For this review, take the finished solid that the model builds, in its own axes (mm). A direction names the side the tool comes from. Coordinates: 2 decimals unless noted, no trailing zeros. Loops run counter-clockwise (first coordinate to the right, second up) from the corner with the lowest first, then second, coordinate; pieces in that order, holes last. Notation, with made-up numbers: (24.5, 18.5) -> (60.5, 18.5) arc R3 ccw to (60.5, 23.5) -> close; hole circle Ø1 at (12, 62.25). An arc over 180 degrees is marked (long way). Use a Markdown table: item, result.
from build123d import *

# Parameters (mm, degrees)
SKETCH1_W            = 20
SKETCH1_H            = 28.7
BOSS_EXTRUDE1_DEPTH  = 17.15
CUT_EXTRUDE1_START   = -1.56
SKETCH2_R            = 7.85
CUT_EXTRUDE1_DEPTH   = 25.58
CUT_EXTRUDE2_DEPTH   = 39.959113
BOSS_EXTRUDE2_DEPTH  = 6.3
M4_CLEARANCE_HOLE1_D = 4.8
CUT_REVOLVE3_START   = -16.206498
CUT_REVOLVE3_DEPTH   = 3.8
CUT_REVOLVE4_START   = -16.206498
CUT_REVOLVE4_DEPTH   = 3.8
SKETCH10_W           = 20
SKETCH10_H           = 3.8
CUT_EXTRUDE3_DEPTH   = 5.3
FILLET1_R            = 2


# Read off the part's stored shape, not the designer's step: Cut-Revolve3, Cut-Revolve4
with BuildPart() as part:
    # Sketch1 → Boss-Extrude1 (new body)
    with BuildSketch(Plane(origin=(0, 0, 0), x_dir=(1, 0, 0), z_dir=(0, 1, 0))):
        with Locations((10, 14.35)):
            Rectangle(SKETCH1_W, SKETCH1_H)
    extrude(amount=BOSS_EXTRUDE1_DEPTH)

    # Sketch2 → Cut-Extrude1 (cut)
    with BuildSketch(Plane.XY.offset(CUT_EXTRUDE1_START)):
        with Locations((10, 17.15)):
            Circle(SKETCH2_R)
    extrude(amount=-CUT_EXTRUDE1_DEPTH, mode=Mode.SUBTRACT)

    # Sketch3 → Cut-Extrude2 (cut, through all)
    with BuildSketch(Plane.XY):
        with BuildLine():
            Line((2.15, 17.15), (17.85, 17.15))
            ThreePointArc((17.85, 17.15), (17.260735, 14.166005), (15.581407, 11.63))
            Line((15.581407, 11.63), (14.85, 11.63))
            Line((14.85, 11.63), (5.15, 11.63))
            Line((5.15, 11.63), (4.418593, 11.63))
            ThreePointArc((4.418593, 11.63), (2.739265, 14.166005), (2.15, 17.15))
        make_face()
    extrude(amount=-CUT_EXTRUDE2_DEPTH, mode=Mode.SUBTRACT)

    # Sketch4 → Boss-Extrude2 (add)
    with BuildSketch(Plane.XZ):
        with BuildLine():
            Line((20, -7.32), (23.289272, -7.32))
            ThreePointArc((23.289272, -7.32), (23.559552, -7.357218), (23.809713, -7.466102))
            Line((23.809713, -7.466102), (28.570441, -10.367714))
            ThreePointArc((28.570441, -10.367714), (28.921906, -10.731939), (29.05, -11.221612))
            Line((29.05, -11.221612), (29.05, -17.478388))
            ThreePointArc((29.05, -17.478388), (28.921906, -17.968061), (28.570441, -18.332286))
            Line((28.570441, -18.332286), (23.809713, -21.233898))
            ThreePointArc((23.809713, -21.233898), (23.559552, -21.342782), (23.289272, -21.38))
            Line((23.289272, -21.38), (20, -21.38))
            Line((20, -21.38), (20, -7.32))
        make_face()
    boss_extrude2 = extrude(amount=-BOSS_EXTRUDE2_DEPTH)

    # Mirror1: Boss-Extrude2 across plane
    add(boss_extrude2.mirror(Plane(origin=(10, 0, 0), x_dir=(0, 0, 1), z_dir=(1, 0, 0))))

    # M4 Clearance Hole1 (through all)
    with Locations(Plane(origin=(0, 6.3, 0), x_dir=(1, 0, 0), z_dir=(0, 1, 0))):
        with Locations((24.1, 14.35), (-4.1, 14.35)):
            Hole(M4_CLEARANCE_HOLE1_D / 2)

    # Cut-Revolve3 outline → Cut-Revolve3 (cut)
    with BuildSketch(Plane.XY.offset(CUT_REVOLVE3_START)):
        with BuildLine():
            Line((0, 10.534858), (0, 2.606187))
            ThreePointArc((0, 2.606187), (2.795508, 1.037341), (5.828669, 0))
            Line((5.828669, 0), (10, 0))
            Line((10, 0), (10, 5.16))
            ThreePointArc((10, 5.16), (4.323533, 6.588853), (0, 10.534858))
        make_face()
    extrude(amount=CUT_REVOLVE3_DEPTH, mode=Mode.SUBTRACT)

    # Cut-Revolve4 outline → Cut-Revolve4 (cut)
    with BuildSketch(Plane.XY.offset(CUT_REVOLVE4_START)):
        with BuildLine():
            ThreePointArc((20, 10.534858), (15.676467, 6.588853), (10, 5.16))
            Line((10, 5.16), (10, 0))
            Line((10, 0), (14.171331, 0))
            ThreePointArc((14.171331, 0), (17.204492, 1.037341), (20, 2.606187))
            Line((20, 2.606187), (20, 10.534858))
        make_face()
    extrude(amount=CUT_REVOLVE4_DEPTH, mode=Mode.SUBTRACT)

    # Sketch10 → Cut-Extrude3 (cut)
    with BuildSketch(Plane.XZ):
        with Locations((10.028669, -14.306498)):
            Rectangle(SKETCH10_W, SKETCH10_H)
    extrude(amount=-CUT_EXTRUDE3_DEPTH, mode=Mode.SUBTRACT)

    # Fillet1
    fillet1_edges = [part.edges().sort_by_distance(p)[0] for p in [
        (0, 8.575, -28.7),
        (20, 8.575, -28.7),
        (20, 8.575, 0),
        (0, 8.575, 0),
    ]]
    fillet(fillet1_edges, radius=FILLET1_R)


solid = part.part
(1) For faces 1 (the face through (-7, 6.3, -14)), 2 (the face through (-2, 3, -7.32)), 3 (the face through (20.029, 3, -14)), 4 (the face through (10, 11.63, -1)), 5 (the face through (22, 3, -7.32)), list the 3-axis set-ups (+Z, -Z, +X, -X, +Y, -Y) from which the entire face can be reached by the end or side of a thin tool; tool diameter is ignored.
Found:
| item | result |
|---|---|
| face 1 | +Z, -Z, -X, +Y |
| face 2 | +Z, -X, +Y, -Y |
| face 3 | -Y |
| face 4 | +Z, -Z, +Y |
| face 5 | +Z, +X, +Y, -Y |
(2) Mouldability with a two-part tool opening along Z and no side actions: class faces 6 (the face through (0.029, 1, -14)), 7 (the face through (29.05, 3, -14)), 8 (the face through (0, 4, -14)), 9 (the face through (-6.16, 3.11, -8.9)) as pulls with the +Z half, pulls with the -Z half, needs draft (parallel to the pull), parting line crosses it, or undercut.
Found:
| item | result |
|---|---|
| face 6 | undercut |
| face 7 | needs draft |
| face 8 | undercut |
| face 9 | pulls with the +Z half |
(3) Take a section at D-D on x = 10. Write out the cut boundary in (y, z).
Found:
| item | result |
|---|---|
| outline | (0, -28.7) -> (11.63, -28.7) -> (11.63, -27.14) -> (9.3, -27.14) -> (9.3, -1.56) -> (11.63, -1.56) -> (11.63, 0) -> (0, 0) -> (0, -12.41) -> (5.3, -12.41) -> (5.3, -16.21) -> (0, -16.21) -> close |
(4) For pin 1 Ø1.8 at (x, z) = (9, -14) entering from -Y; pin 2 Ø5 at (y, z) = (10, -8.5) entering from +X; pin 3 Ø4.5 at (x, z) = (-4.1, -14.35) entering from -Y; pin 4 Ø2 at (y, z) = (15, -4) entering from -X, all flat-tipped, find the tip position at first contact; note any pin that passes through.
Found:
| item | result |
|---|---|
| pin 1 | stops at y = 5.3 |
| pin 2 | stops at x = 20 |
| pin 3 | passes through |
| pin 4 | stops at x = 0 |
(5) Take a section at A-A on y = 4.75. State how many separate pieces and enclosed holes the cut face has, plus the area to 3 significant figures.
Found:
| item | result |
|---|---|
| separate pieces | 1 |
| enclosed holes | 3 |
| area | 676 mm^2 |
(6) Take a section at C-C on y = 14. Write out the cut boundary in (x, z), plus the area to 3 significant figures.
Found:
| item | result |
|---|---|
| outline | (0, -26.7) arc R2 ccw to (2, -28.7) -> (2.81, -28.7) -> (2.81, 0) -> (2, 0) arc R2 ccw to (0, -2) -> close; (17.19, -28.7) -> (18, -28.7) arc R2 ccw to (20, -26.7) -> (20, -2) arc R2 ccw to (18, 0) -> (17.19, 0) -> close |
| area | 158 mm^2 |
(7) For line 1 along X through (y, z) = (4.75, -14.35); line 2 along Z through (x, y) = (14, 4); line 3 along X through (y, z) = (12.25, -6.25), list the stretches that pass through material, from the lowest coordinate up.
Found:
| item | result |
|---|---|
| line 1 | x = -9.05 to -6.5, -1.7 to 0, 20.03 to 21.7, 26.5 to 29.05 |
| line 2 | z = -28.7 to -16.21, -12.41 to 0 |
| line 3 | x = 0 to 3.87, 16.13 to 20 |
